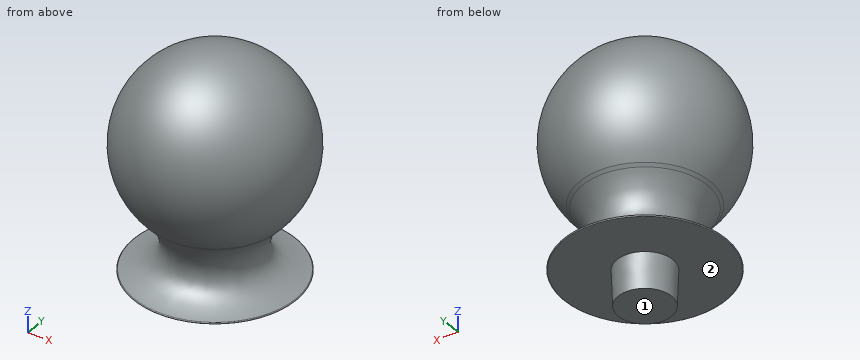
```python
from build123d import *


# Not quite as in the source:
# - a fillet or chamfer that OpenCascade refuses, or shapes differently, is made with other operations: its cross-section is extruded or revolved along the edge and cut away or added


with BuildPart() as f1:
    # F0 (on Front) → F1 (revolve)
    with BuildSketch(Plane.XZ):
        with BuildLine():
            add(Edge.make_bspline(
                [(2.5003758306, 0.0177362721), (2.4404300279, -0.0413985663), (2.3744789771, -0.1082652449), (2.3049510778, -0.1817676763)],
                knots=[0, 0, 0, 0, 0.0510069156, 0.0510069156, 0.0510069156, 0.0510069156], degree=3))
            ThreePointArc((2.5003758306, 0.0177362721), (3.6940969816, 6.8849464932), (-2.1325040052, 10.7104225876))
            Line((-2.1325040052, 10.7104225876), (-2.132504005, -1.9895774124))
            ThreePointArc((-2.132504005, -1.9895774124), (0.2632831128, -1.5202835001), (2.3049510778, -0.1817676763))
        make_face()
        with BuildLine():
            ThreePointArc((2.3049510778, -0.1817676763), (2.4037603545, -0.0830901744), (2.5003758306, 0.0177362721))
            add(Edge.make_bspline(
                [(2.5003758306, 0.0177362721), (2.4404300279, -0.0413985663), (2.3744789771, -0.1082652449), (2.3049510778, -0.1817676763)],
                knots=[0, 0, 0, 0, 0.0510069156, 0.0510069156, 0.0510069156, 0.0510069156], degree=3))
        make_face()
        with BuildLine():
            add(Edge.make_bspline(
                [(2.3049510778, -0.1817676763), (1.9642470512, -0.5419479004), (1.0532611933, -1.6513807021), (1.0539929138, -3.8701076312), (3.2527025422, -4.5295774125), (5.0868722728, -4.5295774125)],
                knots=[0.0510069156, 0.0510069156, 0.0510069156, 0.0510069156, 0.300953508, 0.5847659526, 1, 1, 1, 1], degree=3))
            ThreePointArc((2.3049510778, -0.1817676763), (0.2632831128, -1.5202835001), (-2.132504005, -1.9895774124))
            Line((-2.132504005, -1.9895774124), (-2.1325040049, -4.5295774124))
            Line((-2.1325040049, -4.5295774124), (-0.2275040048, -4.5295774124))
            Line((-0.2275040048, -4.5295774124), (-0.1388052504, -4.5295774124))
            Line((-0.1388052504, -4.5295774124), (5.0868722728, -4.5295774125))
        make_face()
        Polygon((-0.2275040048, -4.5295774124), (-2.1325040049, -4.5295774124), (-2.1325040049, -7.0695774124), (-0.2275040049, -7.0695774124), (-0.1388052504, -4.5295774124), align=None)
    revolve(axis=Axis((-2.132504005, 0, 3.0904225876), (0, 0, -1)))

    # F2: fillet of radius 0.0508 on 1 edges, made by hand

    # F2_s1 → F2_t2 (revolve, cut)
    with BuildSketch(Plane.XZ):
        with BuildLine():
            ThreePointArc((3.6079651255, -4.4285482526), (3.651028038, -4.4825852127), (3.6003709491, -4.5295774123))
            Line((3.6003709491, -4.5295774123), (3.6003709491, -4.5305934123))
            Line((3.6003709491, -4.5305934123), (5.0868722728, -4.5305934125))
            Line((5.0868722728, -4.5305934125), (5.0868722728, -4.5285614125))
            ThreePointArc((5.0868722728, -4.5285614125), (4.3457025483, -4.5054914795), (3.6081170091, -4.4275436694))
            Line((3.6081170091, -4.4275436694), (3.6079651255, -4.4285482526))
        make_face()
    revolve(axis=Axis((-2.1325040049, 0, -4.5295774126), (0, 0, -1)), mode=Mode.SUBTRACT)


solid = f1.part
```
Design review of the part built by this model. Coordinates are the model's own, in mm. Face numbers are marked on the shaded views. A direction names the side the tool comes from. Round coordinates to 2 decimals unless told otherwise and drop trailing zeros. Order: outer loops, then holes, each group sorted by start corner. A loop starts at its lowest first (then second) coordinate and runs counter-clockwise, first axis right, second up. Notation, with made-up numbers: (11.25, -10.5) - (15.25, -10.5) arc R22 cw to (15.25, 23.5) - close; hole circle Ø9 at (42.25, 65.5). An arc over 180 degrees is marked (long way). One line per question, with ' | ' between items.
Item 1: For P1, Ø2, axis at x = 0.5, y = -4.5, coming from the +Z side; P2, Ø6, axis at x = 1.5, y = 1, coming from the +Z side; P3, Ø5, axis at x = 1.5, y = -4.5, coming from the -Z side, all flat-tipped, find the tip position at first contact; note any pin that passes through.
Checks:
P1: z = 9.11 | P2: z = 10.66 | P3: z = -4.53
Item 2: Wall thickness on line 1 (Z direction, x = 0.5, y = 2.75); line 2 (Z direction, x = -4.25, y = 4); line 3 (X direction, y = -2.5, z = -4): over which ranges is each line inside the solid? List them lowest first. Write a range as [from, to].
Checks:
line 1: [-4.53, -3.68], [-0.95, 9.44] | line 2: [-4.53, -4.11], [-0.09, 8.81] | line 3: [-5.61, 1.35]
Item 3: Machinability: for the marked faces 1 and 2, which of the approach directions +Z, -Z, +X, -X, +Y, -Y give a long, thin tool a straight path to every point of the face, cutting with its end or side? Answer none if there is none.
Checks:
face 1: -Z, +X, -X, +Y, -Y | face 2: -Z
Item 4: Take a section at A-A, the plane z = 4. Write out the cut boundary in (x, y), then the cut area to 3 significant figures.
Checks:
outline: circle Ø12.68 at (-2.13, 0) | area: 126 mm²
Item 5: Take a section at B-B, the plane z = 8.5. Write out the cut boundary in (x, y), then the cut area to 3 significant figures.
Checks:
outline: circle Ø9.63 at (-2.13, 0) | area: 72.8 mm²
